```python
from build123d import *

# Parameters (mm, degrees)
SKETCH1_W           = 54.5
SKETCH1_H           = 24.5
BOSS_EXTRUDE1_DEPTH = 2
BOSS_EXTRUDE2_START = -2
SKETCH2_W           = 58.5
SKETCH2_H           = 28.5
SKETCH2_W_2         = 54.5
SKETCH2_H_2         = 24.5
BOSS_EXTRUDE2_DEPTH = 5
CUT_EXTRUDE1_DEPTH  = 33.918459867
FILL_PATTERN1_DEPTH = 2
LPATTERN1_COUNT     = 2
LPATTERN1_PITCH     = 8.5
LPATTERN1_COL_COUNT = 2
LPATTERN1_COL_PITCH = 8.5
SKETCH13_W          = 8.75
SKETCH13_H          = 3
CUT_EXTRUDE2_DEPTH  = 61.417816081
SKETCH34_R          = 2.1
BOSS_EXTRUDE4_DEPTH = 2


# Read off the part's stored shape, not the designer's step: Fill Pattern1
with BuildPart() as part:
    # Sketch1 → Boss-Extrude1 (new body)
    with BuildSketch(Plane(origin=(0, 0, 0), x_dir=(1, 0, 0), z_dir=(0, 1, 0))):
        Rectangle(SKETCH1_W, SKETCH1_H)
    extrude(amount=BOSS_EXTRUDE1_DEPTH)

    # Sketch2 → Boss-Extrude2 (add)
    with BuildSketch(Plane(origin=(0, 2, 0), x_dir=(1, 0, 0), z_dir=(0, 1, 0)).offset(BOSS_EXTRUDE2_START)):
        Rectangle(SKETCH2_W, SKETCH2_H)
        Rectangle(SKETCH2_W_2, SKETCH2_H_2, mode=Mode.SUBTRACT)
    extrude(amount=BOSS_EXTRUDE2_DEPTH)

    # Sketch5 → Cut-Extrude1 (cut, through all)
    with BuildSketch(Plane.XZ):
        with BuildLine():
            Line((-5, 2), (5, 2))
            ThreePointArc((5, 2), (7, 0), (5, -2))
            Line((5, -2), (-5, -2))
            ThreePointArc((-5, -2), (-7, 0), (-5, 2))
        make_face()
    cut_extrude1 = extrude(amount=-CUT_EXTRUDE1_DEPTH, mode=Mode.SUBTRACT)

    # Fill Pattern1 outline → Fill Pattern1 (cut)
    with BuildSketch(Plane(origin=(0, 0, 0), x_dir=(1, 0, 0), z_dir=(0, 1, 0))):
        with BuildLine():
            ThreePointArc((-22, 2), (-24, 0), (-22, -2))
            Line((-22, -2), (-12, -2))
            ThreePointArc((-12, -2), (-10, 0), (-12, 2))
            Line((-12, 2), (-22, 2))
        make_face()
        with BuildLine():
            ThreePointArc((12, 2), (10, 0), (12, -2))
            Line((12, -2), (22, -2))
            ThreePointArc((22, -2), (24, 0), (22, 2))
            Line((22, 2), (12, 2))
        make_face()
        with BuildLine():
            ThreePointArc((-22, 10.5), (-24, 8.5), (-22, 6.5))
            Line((-22, 6.5), (-12, 6.5))
            ThreePointArc((-12, 6.5), (-10, 8.5), (-12, 10.5))
            Line((-12, 10.5), (-22, 10.5))
        make_face()
        with BuildLine():
            ThreePointArc((12, 10.5), (10, 8.5), (12, 6.5))
            Line((12, 6.5), (22, 6.5))
            ThreePointArc((22, 6.5), (24, 8.5), (22, 10.5))
            Line((22, 10.5), (12, 10.5))
        make_face()
        with BuildLine():
            ThreePointArc((-22, -6.5), (-24, -8.5), (-22, -10.5))
            Line((-22, -10.5), (-12, -10.5))
            ThreePointArc((-12, -10.5), (-10, -8.5), (-12, -6.5))
            Line((-12, -6.5), (-22, -6.5))
        make_face()
        with BuildLine():
            ThreePointArc((12, -6.5), (10, -8.5), (12, -10.5))
            Line((12, -10.5), (22, -10.5))
            ThreePointArc((22, -10.5), (24, -8.5), (22, -6.5))
            Line((22, -6.5), (12, -6.5))
        make_face()
    extrude(amount=FILL_PATTERN1_DEPTH, mode=Mode.SUBTRACT)

    # LPattern1: Cut-Extrude1 ×2
    with Locations(*[(0, 0, i * LPATTERN1_PITCH) for i in range(1, LPATTERN1_COUNT)]):
        add(cut_extrude1, mode=Mode.SUBTRACT)

    # LPattern1 col: Cut-Extrude1 ×2
    with Locations(*[(0, 0, -i * LPATTERN1_COL_PITCH) for i in range(1, LPATTERN1_COL_COUNT)]):
        add(cut_extrude1, mode=Mode.SUBTRACT)

    # Sketch13 → Cut-Extrude2 (cut, through all)
    with BuildSketch(Plane(origin=(29.25, 0, 0), x_dir=(0, 0, -1), z_dir=(1, 0, 0))):
        with Locations((-7.875, 3.5)):
            Rectangle(SKETCH13_W, SKETCH13_H)
        with Locations((7.875, 3.5)):
            Rectangle(SKETCH13_W, SKETCH13_H)
    extrude(amount=-CUT_EXTRUDE2_DEPTH, mode=Mode.SUBTRACT)

    # Mirror1: part across plane


with BuildPart() as part_1:
    add(part.part)
    add(part.part.mirror(Plane.XY.offset(13.25)))

    # Sketch34 → Boss-Extrude4 (add)
    with BuildSketch(Plane(origin=(0, 2, 0), x_dir=(1, 0, 0), z_dir=(0, 1, 0))):
        with BuildLine():
            Line((-29.25, 11.400334068), (-38.010329233, 8.719922842))
            ThreePointArc((-38.010329233, 8.719922842), (-40.54977577, 3.399112638), (-35.029778513, 1.328016256))
            Line((-35.029778513, 1.328016256), (-30.75, 3.5))
            Line((-30.75, 3.5), (-29.25, 3.5))
            Line((-29.25, 3.5), (-29.25, 11.400334068))
        make_face()
        with Locations(Location((-36.84, 4.894961472, 0), (0, 0, 270))):
            Circle(SKETCH34_R, mode=Mode.SUBTRACT)
    extrude(amount=-BOSS_EXTRUDE4_DEPTH)


solid = part_1.part
```
Here's how the part is built. I have some questions about the finished solid (model axes, mm). A direction names the side the tool comes from. Give positions to 0.01 mm unless a question says otherwise; leave off trailing zeros. Loops run counter-clockwise (first coordinate to the right, second up) from the corner with the lowest first, then second, coordinate; pieces in that order, holes last. Notation, with made-up numbers: M -26.75,42.5 L 23.25,42.5 A9 ccw 23.25,50.5 Z; hole C 18.5,-22.5 d6. An arc over 180 degrees is marked long. Return JSON: item names as keys, results as strings.
Item 1: Imagine slicing it at B-B on z = 0. List the corners of the cut face in (x, y) for me, then the cut area to 3 significant figures.
A:
{"outline": "M -29.25,0 L -24,0 L -24,2 L -27.25,2 L -27.25,5 L -29.25,5 Z; M -10,0 L -7,0 L -7,2 L -10,2 Z; M 7,0 L 10,0 L 10,2 L 7,2 Z; M 24,0 L 29.25,0 L 29.25,5 L 27.25,5 L 27.25,2 L 24,2 Z", "area": "45.0 mm^2"}
Item 2: Please list where these lines run through material, in increasing order: line 1 (Z direction, x = 10, y = 4.6); line 2 (X direction, y = 0.4, z = 35); line 3 (X direction, y = 1.75, z = 34).
A:
{"line 1": "z = -14.25 to -12.25, 12.25 to 14.25, 38.75 to 40.75", "line 2": "x = -29.25 to -24, -10 to -7, 7 to 10, 24 to 29.25", "line 3": "x = -29.25 to -23.73, -10.27 to -6.73, 6.73 to 10.27, 23.73 to 29.25"}
Item 3: I'm going to push flat-ended pins straight in: pin 1 Ø2.5 at (y, z) = (4, 0) entering from -X; pin 2 Ø7.5 at (x, z) = (-22.5, -4) entering from +Y. Where does each tip first touch, or does it pass through?
A:
{"pin 1": "stops at x = -29.25", "pin 2": "stops at y = 2"}
Item 4: On a 3-axis mill with a long thin cutter (end or side, diameter ignored), from which of +Z, -Z, +X, -X, +Y, -Y can I reach the whole of each face in a straight line? I mean faces 1 (the flat face through (0, 3, 14.25)), 2 (the flat face through (28, 5, 0)), 3 (the flat face through (-27.25, 3, 0)), 4 (the cylindrical face through (7, 1, 18)). Say none if no direction works.
A:
{"face 1": "+X, -X, +Y", "face 2": "+Z, -Z, +X, -X, +Y", "face 3": "+Y", "face 4": "+Y, -Y"}
Item 5: Imagine slicing it at A-A on y = 2.9. List the corners of the cut face in (x, z) for me.
A:
{"outline": "M -29.25,-14.25 L 29.25,-14.25 L 29.25,-12.25 L -29.25,-12.25 Z; M -29.25,-3.5 L -27.25,-3.5 L -27.25,3.5 L -29.25,3.5 Z; M -29.25,12.25 L 29.25,12.25 L 29.25,14.25 L -29.25,14.25 Z; M -29.25,23 L -27.25,23 L -27.25,30 L -29.25,30 Z; M -29.25,38.75 L 29.25,38.75 L 29.25,40.75 L -29.25,40.75 Z; M 27.25,-3.5 L 29.25,-3.5 L 29.25,3.5 L 27.25,3.5 Z; M 27.25,23 L 29.25,23 L 29.25,30 L 27.25,30 Z"}
Item 6: Imagine slicing it at C-C on z = 8.5. List the corners of the cut face in (x, y) for me.
A:
{"outline": "M -29.25,0 L -24,0 L -24,2 L -29.25,2 Z; M -10,0 L -7,0 L -7,2 L -10,2 Z; M 7,0 L 10,0 L 10,2 L 7,2 Z; M 24,0 L 29.25,0 L 29.25,2 L 24,2 Z"}
Item 7: Imagine slicing it at D-D on x = -31.5. List the corners of the cut face in (y, z) for me, then the cut area to 3 significant figures.
A:
{"outline": "M 0,-10.71 L 2,-10.71 L 2,-3.12 L 0,-3.12 Z", "area": "15.2 mm^2"}
Item 8: Thinking about a two-plate mould opening in Z: for faces 5 (the flat face through (0, 3, -12.25)), 6 (the flat face through (-28, 5, 27)), which applies, released by +Z, released by -Z, zero draft, split by the parting line, or undercut?
A:
{"face 5": "undercut", "face 6": "zero draft"}
